Verification items for the finished model (mm, model axes). A direction names the side the tool comes from. Coordinates: 2 decimals unless noted, no trailing zeros. Write each loop counter-clockwise with the first axis right and the second up, starting at its lowest first coordinate (ties: lowest second). Pieces come first, ordered by that corner, then holes. Notation, with made-up numbers: (13.25, 89.5) - (46.25, 89.5) arc R27 cw to (46.25, 124.5) - close; hole circle Ø6 at (21, 48.25). An arc over 180 degrees is marked (long way). Answer as CSV lines item,"result". Start each with the question number.
```python
from build123d import *

# Parameters (mm, degrees)
SKETCH1_R           = 2.75
SKETCH1_R_2         = 2.25
BOSS_EXTRUDE1_DEPTH = 4
BOSS_EXTRUDE2_DEPTH = 3
SKETCH3_W           = 10
SKETCH3_H           = 10
BOSS_EXTRUDE3_DEPTH = 15
SKETCH4_R           = 2.5
CUT_EXTRUDE1_DEPTH  = 72.533209071
CHAMFER1_SIZE       = 0.75


with BuildPart() as part:
    # Sketch1 → Boss-Extrude1 (new body)
    with BuildSketch(Plane(origin=(0, 0, 0), x_dir=(1, 0, 0), z_dir=(0, 1, 0))):
        Polygon((-16.679491924, -30), (16.679491924, -30), (34, 0), (34, 30), (-34, 30), (-34, 0), align=None)
        with Locations(Location((-19, 22.5, 0), (0, 0, 270))):
            Circle(SKETCH1_R, mode=Mode.SUBTRACT)
        with Locations(Location((19, 22.5, 0), (0, 0, 270))):
            Circle(SKETCH1_R, mode=Mode.SUBTRACT)
        with Locations(Location((0, -25, 0), (0, 0, 270))):
            Circle(SKETCH1_R, mode=Mode.SUBTRACT)
        with Locations(Location((-29, 15, 0), (0, 0, 270))):
            Circle(SKETCH1_R_2, mode=Mode.SUBTRACT)
        with Locations(Location((29, 15, 0), (0, 0, 270))):
            Circle(SKETCH1_R_2, mode=Mode.SUBTRACT)
        with Locations(Location((0, -15, 0), (0, 0, 270))):
            Circle(SKETCH1_R_2, mode=Mode.SUBTRACT)
    extrude(amount=BOSS_EXTRUDE1_DEPTH)

    # Sketch2 → Boss-Extrude2 (add)
    with BuildSketch(Plane(origin=(0, 4, 0), x_dir=(1, 0, 0), z_dir=(0, 1, 0))):
        Polygon((-26.589820012, -12.834808232), (-24.089671912, -17.165191768), (0, -2.905179879), (24.089671912, -17.165191768), (26.589820012, -12.834808232), (2.5, 1.425291326), (2.5, 30), (-2.5, 30), (-2.5, 1.425291326), align=None)
    extrude(amount=BOSS_EXTRUDE2_DEPTH)

    # Sketch3 → Boss-Extrude3 (add)
    with BuildSketch(Plane(origin=(0, 4, 0), x_dir=(1, 0, 0), z_dir=(0, 1, 0))):
        with Locations((-29, 25)):
            Rectangle(SKETCH3_W, SKETCH3_H)
        with Locations((29, 25)):
            Rectangle(SKETCH3_W, SKETCH3_H)
    extrude(amount=BOSS_EXTRUDE3_DEPTH)

    # Sketch4 → Cut-Extrude1 (cut, through all)
    with BuildSketch(Plane(origin=(0, 0, -30), x_dir=(-1, 0, 0), z_dir=(0, 0, -1))):
        with Locations((-29, 13)):
            Circle(SKETCH4_R)
        with Locations((29, 13)):
            Circle(SKETCH4_R)
    extrude(amount=-CUT_EXTRUDE1_DEPTH, mode=Mode.SUBTRACT)

    # Chamfer1
    chamfer1_edges = [part.edges().sort_by_distance(p)[0] for p in [
        (-19, 4, -25.25),
        (19, 4, -25.25),
        (0, 4, 22.25),
    ]]
    chamfer(chamfer1_edges, length=CHAMFER1_SIZE)


solid = part.part
```
1. Access from +Z, -Z, +X, -X, +Y, -Y to the whole of each face (thin tool, end or side, straight path). Record for faces 1 (the face through (11.876, 5.479, 9.935)), 2 (the face through (0, 2, 30)).
2. Cross-section at B-B (y = 1.75). Record the cut outline in (x, z), and give its area (3 significant figures).
3. Scan lines: line 1 along X through (y, z) = (1.6, -22.5); line 2 along X through (y, z) = (3.05, -15); line 3 along Y through (x, z) = (-28, -19.5). Record each from-to range of solid material in increasing order. Write a range as from..to.
4. Depth check by flat-ended pin: P1, Ø10, axis at y = 14.5, z = 10.5, coming from the +X side; P2, Ø5, axis at y = 4, z = 22, coming from the -X side; P3, Ø8, axis at x = -6.5, z = 23, coming from the +Y side; P4, Ø1.5, axis at y = 6, z = -9, coming from the +X side. Enter the tip coordinate at first touch or a pass-through.
5. Cross-section at A-A (z = -22.5). Record the cut outline in (x, y), and give its area (3 significant figures).
6. Cross-section at C-C (x = -29). Record the cut outline in (y, z), and give its area (3 significant figures).
7. Draft check along X on faces 3 (the face through (-34, 7, -21)), 4 (the face through (2.5, 5, -16)), 5 (the face through (-18, 4, -9)), 6 (the face through (0, 0, 0)). Enter one of: pulls with the +X half, pulls with the -X half, needs draft (parallel to the pull), parting line crosses it, or undercut.
8. Cross-section at D-D (z = 15). Record the cut outline in (x, y).
Completed:
1,face 1,"+Z, +Y"
1,face 2,"+Z, +X, -X, +Y, -Y"
2,outline,"(-34, -30) - (34, -30) - (34, 0) - (16.68, 30) - (-16.68, 30) - (-34, 0) - close; hole circle Ø4.5 at (-29, -15); hole circle Ø5.5 at (-19, -22.5); hole circle Ø5.5 at (0, 25); hole circle Ø4.5 at (0, 15); hole circle Ø5.5 at (19, -22.5); hole circle Ø4.5 at (29, -15)"
2,area,"3,440 mm2"
3,line 1,"x = -34..-21.75, -16.25..16.25, 21.75..34"
3,line 2,"x = -34..-31.25, -26.75..26.75, 31.25..34"
3,line 3,"y = 0..4"
4,P1,"passes through"
4,P2,"stops at x = -22.74"
4,P3,"stops at y = 4"
4,P4,"stops at x = 2.5"
5,outline,"(-34, 0) - (-21.75, 0) - (-21.75, 3.25) - (-22.5, 4) - (-24, 4) - (-24, 19) - (-34, 19) - close; (-16.25, 0) - (16.25, 0) - (16.25, 3.25) - (15.5, 4) - (2.5, 4) - (2.5, 7) - (-2.5, 7) - (-2.5, 4) - (-15.5, 4) - (-16.25, 3.25) - close; (21.75, 0) - (34, 0) - (34, 19) - (24, 19) - (24, 4) - (22.5, 4) - (21.75, 3.25) - close; hole circle Ø5 at (-29, 13); hole circle Ø5 at (29, 13)"
5,area,"503 mm2"
6,outline,"(0, -30) - (10.5, -30) - (10.5, -20) - (4, -20) - (4, -17.25) - (0, -17.25) - close; (0, -12.75) - (4, -12.75) - (4, 8.66) - (0, 8.66) - close; (15.5, -30) - (19, -30) - (19, -20) - (15.5, -20) - close"
6,area,"237 mm2"
7,face 3,"pulls with the -X half"
7,face 4,"undercut"
7,face 5,"undercut"
7,face 6,"needs draft"
8,outline,"(-25.34, 0) - (-2.25, 0) - (-2.25, 4) - (-20.43, 4) - (-20.43, 7) - (-25.34, 7) - close; (2.25, 0) - (25.34, 0) - (25.34, 7) - (20.43, 7) - (20.43, 4) - (2.25, 4) - close"
